Work out the finished part from the listing and answer in its coordinate system (mm). A direction names the side the tool comes from. Round coordinates to 2 decimals unless told otherwise and drop trailing zeros. Write each loop counter-clockwise with the first axis right and the second up, starting at its lowest first coordinate (ties: lowest second). Pieces come first, ordered by that corner, then holes. Notation, with made-up numbers: (77, 85.5) -> (112, 85.5) arc R7 cw to (112, 96.5) -> close; hole circle Ø4 at (-28, 8). An arc over 180 degrees is marked (long way). Answer as a JSON object with one key per item and string values. Group by question number.
from build123d import *

# Parameters (mm, degrees)
MAIN_DEPTH         = 5
WINDOWSLOT1_DEPTH  = 2
SKETCH6_R          = 1.25
CUT_EXTRUDE2_DEPTH = 5
LPATTERN1_COUNT    = 5
LPATTERN1_PITCH    = 10
SKETCH7_R          = 3.5
CUT_EXTRUDE4_DEPTH = 1.5


with BuildPart() as part:
    # Sketch1 → Main (new body, symmetric)
    with BuildSketch(Plane.XY):
        Polygon((-25, -25), (25, 25), (25, 17), (-17, -25), align=None)
    extrude(amount=MAIN_DEPTH, both=True)

    # Sketch4 → WindowSlot1 (cut)
    with BuildSketch(Plane.XY.offset(5)):
        Polygon((25, 22.171572875), (-22.171572875, -25), (-18.636038969, -25), (25, 18.636038969), align=None)
    windowslot1 = extrude(amount=-WINDOWSLOT1_DEPTH, mode=Mode.SUBTRACT)

    # Mirror1: WindowSlot1 across plane
    add(windowslot1.mirror(Plane.XY), mode=Mode.SUBTRACT)

    # Sketch6 → Cut-Extrude2 (cut)
    with BuildSketch(Plane(origin=(4, -4, 0), x_dir=(0, 0, 1), z_dir=(-0.707106781, 0.707106781, 0))):
        with Locations((0, 20)):
            Circle(SKETCH6_R)
    cut_extrude2 = extrude(amount=CUT_EXTRUDE2_DEPTH, mode=Mode.SUBTRACT)

    # LPattern1: Cut-Extrude2 ×5
    with Locations(*[Vector(-0.707106781, -0.707106781, 0) * (i * LPATTERN1_PITCH) for i in range(1, LPATTERN1_COUNT)]):
        add(cut_extrude2, mode=Mode.SUBTRACT)

    # Sketch7 → Cut-Extrude4 (cut)
    with BuildSketch(Plane(origin=(0, 0, 0), x_dir=(0, 0, 1), z_dir=(-0.707106781, 0.707106781, 0))):
        with Locations((0, 20)):
            Circle(SKETCH7_R)
        with Locations((0, -20)):
            Circle(SKETCH7_R)
    extrude(amount=-CUT_EXTRUDE4_DEPTH, mode=Mode.SUBTRACT)


solid = part.part
1) Straight lines are drawn through the part: L1, parallel to Y at x = 8.5, z = 4.5; L2, parallel to Y at x = -15, z = 3.75; L3, parallel to Z at x = 1, y = -4. For each, find the intervals that lie inside material, in ascending order.
2) A cutting plane is placed at A-A on z = 0.5. State how many separate pieces and enclosed holes the cut face has, plus the area to 3 significant figures.
3) For a pull along X with two mould halves and no side action, classify faces 5 (the face through (4, -4, 2)), 6 (the face through (2.877, -3.487, 4.014)), 7 (the face through (-21, -25, 0)) as released by +X, released by -X, zero draft, split by the parting line, or undercut.
4) A cutting plane is placed at B-B on y = -20.5. Determine the outline of the cut face in (x, z).
5) A tool of negligible diameter and unlimited length cuts with its end or side. For faces 1 (the face through (2.877, -3.487, -4.014)), 2 (the face through (1.744, -1.084, 4.014)), 3 (the face through (0, -2, -5)), 4 (the face through (-6.59, -7.52, -0.02)), from which of +Z, -Z, +X, -X, +Y, -Y can it reach the whole face along a straight path? Write none if from no direction.
6) Each of these flat-tipped pins is pushed along its axis until it touches: P1, Ø2, axis at y = 20, z = -2.5, coming from the -X side; P2, Ø3, axis at y = 10.5, z = 2.5, coming from the -X side; P3, Ø3, axis at x = 13, z = 2, coming from the -Y side; P4, Ø14, axis at x = -3.5, y = -7, coming from the -Z side. Where does it stop, or does it pass through?
Established:
{
 "1": {"L1": "y = 0.5 to 2.14, 5.67 to 8.5", "L2": "y = -23 to -21.36, -17.83 to -15", "L3": "z = -3 to 3"},
 "2": {"separate pieces": "3", "enclosed holes": "0", "area": "294 mm²"},
 "3": {"face 5": "released by +X", "face 6": "undercut", "face 7": "zero draft"},
 "4": {"outline": "(-20.5, -5) -> (-17.67, -5) -> (-17.67, -3) -> (-14.14, -3) -> (-14.14, -5) -> (-12.5, -5) -> (-12.5, 5) -> (-14.14, 5) -> (-14.14, 3) -> (-17.67, 3) -> (-17.67, 5) -> (-20.5, 5) -> close"},
 "5": {"face 1": "-Z", "face 2": "+Z", "face 3": "-Z, +X, -X, +Y, -Y", "face 4": "none"},
 "6": {"P1": "stops at x = 19", "P2": "stops at x = 9", "P3": "stops at y = 3.5", "P4": "stops at z = -5"}
}
